Model file for the job. Use its own axes, mm. A direction names the side the tool comes from. Give positions to 0.01 mm unless a question says otherwise; leave off trailing zeros. Order: outer loops, then holes, each group sorted by start corner. A loop starts at its lowest first (then second) coordinate and runs counter-clockwise, first axis right, second up. Notation, with made-up numbers: (-10, -1.5) - (22, -1.5) arc R4 ccw to (22, 4.5) - close; hole circle Ø3 at (-38, 71.25). An arc over 180 degrees is marked (long way). Use CSV: the item, a comma, the result in double quotes. Start each with the question number.
(1) Probe L1, parallel to Y at x = 3, z = 4.5; L2, parallel to Z at x = 0.5, y = 8.5; L3, parallel to Y at x = 2.5, z = 5.25. List the from-to ranges inside material, lowest first.
(2) Band-saw the part on C-C, the plane z = 5.5. Give the cut face in (x, y).
(3) Band-saw the part on D-D, the plane y = 5.75. Give the cut face in (x, z), then the cut area to 3 significant figures.
(4) Tool access for faces 1 (the cylindrical face through (4, 15, 7)), 2 (the flat face through (4, 9, 4)), 3 (the flat face through (5.5, 2, 2)): list every direction of +Z, -Z, +X, -X, +Y, -Y with a clear straight run to the whole face (end or side of a thin tool).
(5) Drop flat-ended pins along their axis: pin 1 Ø1.6 at (x, y) = (7.5, 16) entering from +Z; pin 2 Ø0.5 at (x, y) = (2.5, 2.5) entering from -Z; pin 3 Ø0.6 at (x, y) = (3.5, 1.5) entering from -Z. Give the stop position or say it passes through.
(6) Pull direction X, two halves, no side cores. Call faces 4 (the flat face through (5, 8.9, 3.5)), 5 (the flat face through (4, 4, 2)), 6 (the flat face through (2, 9, 3)): +X half, -X half, draft (parallel to the pull), parting line (faces both ways), or undercut.
Autodesk Fusion 360 part; units mm, degrees
sketch "Sketch1" plane through (0, 0, 0) normal (0, 1, 0) x (1, 0, 0)
  line L0 (0, 0) -> (0, -5)
  line L1 (0, -5) -> (8, -5)
  line L2 (8, -5) -> (8, 0)
  line L3 (8, 0) -> (6, 0)
  line L4 (6, 0) -> (6, -2)
  line L5 (6, -2) -> (5, -2)
  line L6 (5, -2) -> (5, -4)
  line L7 (5, -4) -> (3, -4)
  line L8 (3, -4) -> (3, -2)
  line L9 (3, -2) -> (2, -2)
  line L10 (2, -2) -> (2, 0)
  line L11 (2, 0) -> (0, 0)
  dimension "d1" = 8
  dimension "d2" = 2
extrude "Extrude1" add sketch "Sketch1" along normal blind 1
sketch "Sketch2" plane through (8, 0, 0) normal (1, 0, 0) x (0, 1, 0)
  line L0 (0, 5) -> (0, 0)
  line L1 (0, 0) -> (1, 0)
  line L2 (1, 0) -> (1, 5)
  line L3 (1, 5) -> (0, 5)
  line L4 (1, 5) -> (4, 5)
  line L5 (4, 5) -> (4, 8)
  arc A0 (4, 8) -> (1, 5) centre (4, 5) ccw
  line L6 (4, 5) -> (4, 0)
  line L7 (4, 0) -> (1, 0)
  dimension "d5" = 3
  dimension "d6" = 3
extrude "Extrude2" add sketch "Sketch2" against normal blind 8 contours L2 L4 L6 L7 | L4 L5 A0
extrude "Extrude3" cut 1 faces at (4.3333, 1, 0.6667) along direction (0, 1, 0) blind 4.5
sketch "Sketch3" plane through (0, 4, 0) normal (0, 1, 0) x (-1, 0, 0)
  line L0 (-2, 2) -> (-2, 0)
  line L1 (-2, 0) -> (0, 0)
  line L2 (0, 0) -> (0, 8)
  line L3 (0, 8) -> (-8, 8)
  line L4 (-8, 8) -> (-8, 0)
  line L5 (-8, 0) -> (-6, 0)
  line L6 (-6, 0) -> (-6, 2)
  line L7 (-6, 2) -> (-5, 2)
  line L8 (-5, 2) -> (-5, 4)
  line L9 (-5, 4) -> (-3, 4)
  line L10 (-3, 4) -> (-3, 2)
  line L11 (-3, 2) -> (-2, 2)
  line L12 (-8, 0) -> (-8, 3)
  line L13 (-8, 3) -> (-5, 3)
  line L14 (-5, 3) -> (-5, 4)
  line L15 (-3, 4) -> (-3, 3)
  line L16 (-3, 3) -> (0, 3)
  line L17 (-3, 4) -> (-5, 4)
  line L18 (0, 3) -> (0, 0)
  line L19 (-8, 0) -> (0, 0)
  dimension "d11" = 3
  dimension "d12" = 3
extrude "Extrude4" add sketch "Sketch3" along normal blind 10 contours L0 L1 L2 L10 L11 L16 L18 L19 | L0 L6 L7 L8 L9 L10 L11 L14 L15 L17 L19 | L4 L5 L6 L7 L8 L12 L13 L19
sketch "Sketch4" plane through (0, 14, 0) normal (0, 1, 0) x (-1, 0, 0)
  line L0 (-8, 3) -> (-8, 0)
  line L1 (-8, 0) -> (0, 0)
  line L2 (0, 0) -> (0, 3)
  line L3 (0, 3) -> (-3, 3)
  line L4 (-3, 3) -> (-3, 4)
  line L5 (-3, 4) -> (-5, 4)
  line L6 (-5, 4) -> (-5, 3)
  line L7 (-5, 3) -> (-8, 3)
  line L8 (-8, 0) -> (-8, 5)
  line L9 (-8, 5) -> (-6, 5)
  line L10 (-6, 5) -> (-4, 5)
  arc A0 (-2, 5) -> (-6, 5) centre (-4, 5) ccw
  line L11 (-2, 5) -> (0, 5)
  line L12 (0, 5) -> (0, 0)
  dimension "d15" = 5
  dimension "d16" = 2
extrude "Extrude5" add sketch "Sketch4" along normal blind 3
Answer block:
1,L1,"y = 0 to 4, 14 to 17"
1,L2,"z = 0 to 3"
1,L3,"y = 1.01 to 4, 14 to 17"
2,outline,"(0, 1.04) - (8, 1.04) - (8, 4) - (0, 4) - close; (2.06, 14) - (5.94, 14) - (5.94, 17) - (2.06, 17) - close"
3,outline,"(0, 0) - (8, 0) - (8, 3) - (5, 3) - (5, 4) - (3, 4) - (3, 3) - (0, 3) - close"
3,area,"26.0 mm2"
4,face 1,"+Z, +Y"
4,face 2,"+Z, +X, -X"
4,face 3,"-Z, -Y"
5,pin 1,"stops at z = 5"
5,pin 2,"stops at z = 2"
5,pin 3,"stops at z = 4"
6,face 4,"+X half"
6,face 5,"undercut"
6,face 6,"draft"
